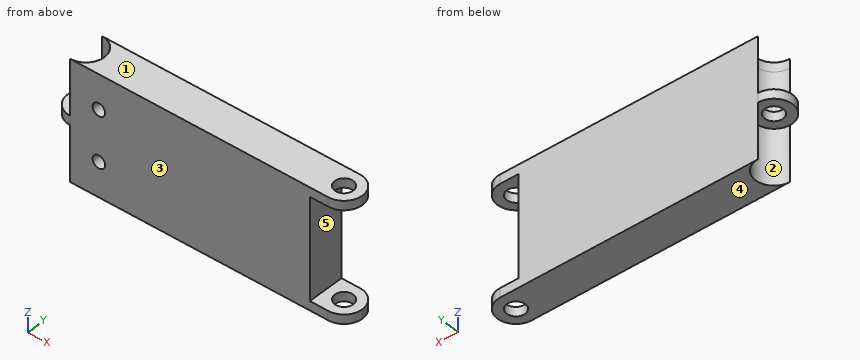
from build123d import *

# Parameters (mm, degrees)
F0_R      = 1.6
F1_DEPTH  = 1.6
F4_DEPTH  = 8
F5_R      = 1.6
F6_DEPTH  = 1.6
F8_DEPTH  = 8
F9_R      = 1.6
F10_DEPTH = 1.6
F12_D     = 2.2
F12_DEPTH = 2.4
F12_TIP   = 0.6609466809


with BuildPart() as f1:
    # F0 (on Top) → F1 (new body)
    with BuildSketch(Plane.XY):
        with BuildLine():
            Line((19.3, 3.2), (-22.5, 3.2))
            ThreePointArc((-22.5, 3.2), (-20.2372583002, 2.2627416998), (-19.3, 0))
            ThreePointArc((-19.3, 0), (-20.2372583002, -2.2627416998), (-22.5, -3.2))
            Line((-22.5, -3.2), (19.3, -3.2))
            Line((19.3, -3.2), (19.3, 0))
            Line((19.3, 0), (19.3, 3.2))
        make_face()
        with BuildLine():
            Line((22.5, 3.2), (19.3, 3.2))
            Line((19.3, 3.2), (19.3, 0))
            ThreePointArc((19.3, 0), (20.2372583002, 2.2627416998), (22.5, 3.2))
        make_face()
        with BuildLine():
            ThreePointArc((25.7, 0), (24.7627416998, 2.2627416998), (22.5, 3.2))
            ThreePointArc((22.5, 3.2), (20.2372583002, 2.2627416998), (19.3, 0))
            ThreePointArc((19.3, 0), (20.2372583002, -2.2627416998), (22.5, -3.2))
            ThreePointArc((22.5, -3.2), (24.7627416998, -2.2627416998), (25.7, 0))
        make_face()
        with Locations((22.5, 0)):
            Circle(F0_R, mode=Mode.SUBTRACT)
        with BuildLine():
            Line((19.3, 0), (19.3, -3.2))
            Line((19.3, -3.2), (22.5, -3.2))
            ThreePointArc((22.5, -3.2), (20.2372583002, -2.2627416998), (19.3, 0))
        make_face()
    extrude(amount=F1_DEPTH)

    # F3 (on offset) → F4 (join)
    with BuildSketch(Plane.XY.offset(1.6)):
        with BuildLine():
            ThreePointArc((-22.5, 3.2), (-20.2372583002, 2.2627416998), (-19.3, 0))
            ThreePointArc((-19.3, 0), (-20.2372583002, -2.2627416998), (-22.5, -3.2))
            Line((-22.5, -3.2), (19.3, -3.2))
            Line((19.3, -3.2), (19.3, 0))
            Line((19.3, 0), (19.3, 3.2))
            Line((19.3, 3.2), (-22.5, 3.2))
        make_face()
    extrude(amount=F4_DEPTH)

    # F5 (on face) → F6 (join)
    with BuildSketch(Plane.XY.offset(9.6)):
        with BuildLine():
            Line((-22.5, -3.2), (19.3, -3.2))
            Line((19.3, -3.2), (19.3, 3.2))
            Line((19.3, 3.2), (-22.5, 3.2))
            ThreePointArc((-22.5, 3.2), (-20.2372583002, 2.2627416998), (-19.3, 0))
            ThreePointArc((-19.3, 0), (-20.2372583002, -2.2627416998), (-22.5, -3.2))
        make_face()
        with BuildLine():
            ThreePointArc((-22.5, 3.2), (-25.7, 0), (-22.5, -3.2))
            ThreePointArc((-22.5, -3.2), (-20.2372583002, -2.2627416998), (-19.3, 0))
            ThreePointArc((-19.3, 0), (-20.2372583002, 2.2627416998), (-22.5, 3.2))
        make_face()
        with Locations((-22.5, 0)):
            Circle(F5_R, mode=Mode.SUBTRACT)
    extrude(amount=F6_DEPTH)

    # F7 (on face) → F8 (join)
    with BuildSketch(Plane.XY.offset(11.2)):
        with BuildLine():
            Line((-22.5, -3.2), (19.3, -3.2))
            Line((19.3, -3.2), (19.3, 0))
            Line((19.3, 0), (19.3, 3.2))
            Line((19.3, 3.2), (-22.5, 3.2))
            ThreePointArc((-22.5, 3.2), (-20.2372583002, 2.2627416998), (-19.3, 0))
            ThreePointArc((-19.3, 0), (-20.2372583002, -2.2627416998), (-22.5, -3.2))
        make_face()
    extrude(amount=F8_DEPTH)

    # F9 (on face) → F10 (join)
    with BuildSketch(Plane.XY.offset(19.2)):
        with BuildLine():
            Line((19.3, -3.2), (19.3, 0))
            Line((19.3, 0), (19.3, 3.2))
            Line((19.3, 3.2), (-22.5, 3.2))
            ThreePointArc((-22.5, 3.2), (-19.3, 0), (-22.5, -3.2))
            Line((-22.5, -3.2), (19.3, -3.2))
        make_face()
        with BuildLine():
            ThreePointArc((19.3, 0), (20.2372583002, 2.2627416998), (22.5, 3.2))
            Line((22.5, 3.2), (19.3, 3.2))
            Line((19.3, 3.2), (19.3, 0))
        make_face()
        with BuildLine():
            ThreePointArc((22.5, -3.2), (24.7627416998, -2.2627416998), (25.7, 0))
            ThreePointArc((25.7, 0), (24.7627416998, 2.2627416998), (22.5, 3.2))
            ThreePointArc((22.5, 3.2), (20.2372583002, 2.2627416998), (19.3, 0))
            ThreePointArc((19.3, 0), (20.2372583002, -2.2627416998), (22.5, -3.2))
        make_face()
        with Locations((22.5, 0)):
            Circle(F9_R, mode=Mode.SUBTRACT)
        with BuildLine():
            Line((19.3, -3.2), (22.5, -3.2))
            ThreePointArc((22.5, -3.2), (20.2372583002, -2.2627416998), (19.3, 0))
            Line((19.3, 0), (19.3, -3.2))
        make_face()
    extrude(amount=F10_DEPTH)

    # F12
    with Locations(Plane.XZ.offset(3.2)):
        with Locations((-17.5, 14.8), (-17.5, 6)):
            Hole(F12_D / 2, depth=F12_DEPTH)
            with Locations((0, 0, -(F12_DEPTH + F12_TIP / 2))):  # 118° drill point
                Cone(0, F12_D / 2, F12_TIP, mode=Mode.SUBTRACT)


solid = f1.part
Work out the finished part from the listing and answer in its coordinate system (mm). Face numbers are marked on the shaded views. A direction names the side the tool comes from. Round coordinates to 2 decimals unless told otherwise and drop trailing zeros. Write each loop counter-clockwise with the first axis right and the second up, starting at its lowest first coordinate (ties: lowest second). Pieces come first, ordered by that corner, then holes. Notation, with made-up numbers: (-24.5, 75) -> (-6.5, 75) arc R21 cw to (-6.5, 88) -> close; hole circle Ø3 at (28.5, -0.5). An arc over 180 degrees is marked (long way). Answer as CSV lines item,"result". Start each with the question number.
(1) The mould has two halves that part along Y. Classify the marked faces 1, 2 and 3: +Y half, -Y half, draft (parallel to the pull), parting line (faces both ways), or undercut.
(2) Each of these flat-tipped pins is pushed along its axis until it touches: pin 1 (1.8 mm diameter, centred on x = -17.5, z = 14.8, fed in from -Y); pin 2 (3 mm diameter, centred on x = -23.5, y = -0.5, fed in from +Z). Where does it stop, or does it pass through?
(3) Find the intervals of material crossed by probe 1 along Z at (x, y) = (-17.5, -1.3); probe 2 along Y at (x, z) = (-22.5, 10.05); probe 3 along Z at (x, y) = (20, -1), in increasing order.
(4) A tool of negligible diameter and unlimited length cuts with its end or side. For the marked faces 4 and 5, from which of +Z, -Z, +X, -X, +Y, -Y can it reach the whole face along a straight path? Write none if from no direction.
(5) The part is cut by section C-C, the plane z = 13. Give the vertices of the cut face in (x, y), then the cut area to 3 significant figures.
(6) The part is cut by section A-A, the plane z = 10.75. Give the vertices of the cut face in (x, y).
(7) The part is cut by section B-B, the plane y = -2.75. Give the vertices of the cut face in (x, z), then the cut area to 3 significant figures.
Output values:
1,face 1,"draft"
1,face 2,"undercut"
1,face 3,"-Y half"
2,pin 1,"stops at y = -0.68"
2,pin 2,"stops at z = 11.2"
3,probe 1,"z = 0 to 4.9, 7.1 to 13.7, 15.9 to 20.8"
3,probe 2,"y = -3.2 to -1.6, 1.6 to 3.2"
3,probe 3,"z = 0 to 1.6, 19.2 to 20.8"
4,face 4,"-Z, +X, -X, +Y, -Y"
4,face 5,"+X, +Y, -Y"
5,outline,"(-22.5, -3.2) -> (19.3, -3.2) -> (19.3, 3.2) -> (-22.5, 3.2) arc R3.2 cw to start"
5,area,"251 mm²"
6,outline,"(-22.5, -3.2) -> (19.3, -3.2) -> (19.3, 3.2) -> (-22.5, 3.2) arc R3.2 ccw to start; hole circle Ø3.2 at (-22.5, 0)"
7,outline,"(-24.14, 9.6) -> (-20.86, 9.6) -> (-20.86, 0) -> (24.14, 0) -> (24.14, 1.6) -> (19.3, 1.6) -> (19.3, 19.2) -> (24.14, 19.2) -> (24.14, 20.8) -> (-20.86, 20.8) -> (-20.86, 11.2) -> (-24.14, 11.2) -> close; hole circle Ø2.2 at (-17.5, 6); hole circle Ø2.2 at (-17.5, 14.8)"
7,area,"849 mm²"
